Here's how the part is built. I have some questions about the finished solid (model axes, mm). Face numbers are marked on the shaded views. A direction names the side the tool comes from. Round coordinates to 2 decimals unless told otherwise and drop trailing zeros. Order: outer loops, then holes, each group sorted by start corner. A loop starts at its lowest first (then second) coordinate and runs counter-clockwise, first axis right, second up. Notation, with made-up numbers: (23.25, 85) -> (36.25, 85) arc R16 ccw to (36.25, 91) -> close; hole circle Ø3 at (35.5, 74.25). An arc over 180 degrees is marked (long way). One line per item, written item: value.
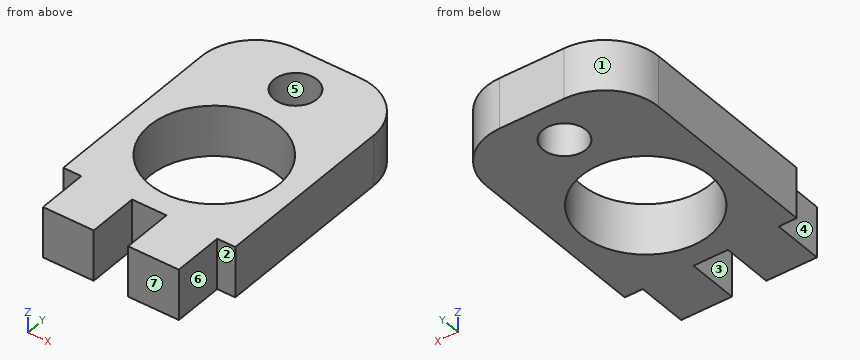
```python
from build123d import *

# Parameters (mm, degrees)
SKETCH1_R           = 3.81
SKETCH1_R_2         = 1.27
BOSS_EXTRUDE1_DEPTH = 2.9972
FILLET1_R           = 3.175


with BuildPart() as part:
    # Sketch1 → Boss-Extrude1 (new body)
    with BuildSketch(Plane.XY):
        Polygon((0, 0), (1.0668, 0), (1.0668, -2.9972), (4.064, -2.9972), (4.064, 0), (6.096, 0), (6.096, -2.9972), (9.0932, -2.9972), (9.0932, 0), (10.16, 0), (10.16, 13.97), (0, 13.97), align=None)
        with Locations(Location((5.08, 5.08, 0), (0, 0, 180))):
            Circle(SKETCH1_R, mode=Mode.SUBTRACT)
        with Locations(Location((5.08, 11.43, 0), (0, 0, 180))):
            Circle(SKETCH1_R_2, mode=Mode.SUBTRACT)
    extrude(amount=BOSS_EXTRUDE1_DEPTH)

    # Fillet1
    fillet1_edges = [part.edges().sort_by_distance(p)[0] for p in [
        (0, 13.97, 1.4986),
        (10.16, 13.97, 1.4986),
    ]]
    fillet(fillet1_edges, radius=FILLET1_R)


solid = part.part
```
Q1. I want a section at C-C on z = 1.75. Write out the boundary of the cut face in (x, y) (3 decimals).
Answers:
outline: (0, 0) -> (1.067, 0) -> (1.067, -2.997) -> (4.064, -2.997) -> (4.064, 0) -> (6.096, 0) -> (6.096, -2.997) -> (9.093, -2.997) -> (9.093, 0) -> (10.16, 0) -> (10.16, 10.795) arc R3.175 ccw to (6.985, 13.97) -> (3.175, 13.97) arc R3.175 ccw to (0, 10.795) -> close; hole circle Ø7.62 at (5.08, 5.08); hole circle Ø2.54 at (5.08, 11.43)
Q2. I want a section at D-D on x = 5. Write out the boundary of the cut face in (y, z).
Answers:
outline: (0, 0) -> (1.27, 0) -> (1.27, 3) -> (0, 3) -> close; (8.89, 0) -> (10.16, 0) -> (10.16, 3) -> (8.89, 3) -> close; (12.7, 0) -> (13.97, 0) -> (13.97, 3) -> (12.7, 3) -> close
Q3. If we mould it in two halves opening along X, with no side actions, what happens to the marked faces 5, 6 and 7? For each: pulls with the +X half, pulls with the -X half, needs draft (parallel to the pull), parting line crosses it, or undercut.
Answers:
face 5: undercut
face 6: pulls with the +X half
face 7: needs draft
Q4. I want a section at A-A on y = -1.5. Write out the boundary of the cut face in (x, z), then the cut area to 3 significant figures.
Answers:
outline: (1.07, 0) -> (4.06, 0) -> (4.06, 3) -> (1.07, 3) -> close; (6.1, 0) -> (9.09, 0) -> (9.09, 3) -> (6.1, 3) -> close
area: 18.0 mm2
Q5. Which directions (+Z, -Z, +X, -X, +Y, -Y) give clear straight access to the entire face, cutting with the end or side of a thin tool? Please do the marked faces 1, 2, 3 and 4.
Answers:
face 1: +Z, -Z, -X, +Y
face 2: +Z, -Z, +X, -Y
face 3: +Z, -Z, -Y
face 4: +Z, -Z, -X, -Y
Q6. I want a section at B-B on x = 7.5. Write out the boundary of the cut face in (y, z).
Answers:
outline: (-3, 0) -> (2.14, 0) -> (2.14, 3) -> (-3, 3) -> close; (8.02, 0) -> (13.93, 0) -> (13.93, 3) -> (8.02, 3) -> close
Q7. For P1, Ø1, axis at x = 5, z = 2, coming from the -Y side; P2, Ø0.9, axis at y = -2, z = 2, coming from the +X side; P3, Ø6, axis at x = 5.08, y = 5.08, coming from the -Z side; P4, Ø0.9, axis at y = -2, z = 1.5, coming from the -X side, each with a flat end and sliding along its axis, tell me the tip position at first contact or that it passes through.
Answers:
P1: y = 0
P2: x = 9.09
P3: through
P4: x = 1.07
Q8. I need wall thicknesses on line 1 along Y through (x, z) = (5.08, 1.1); line 2 along Y through (x, z) = (4, 1.25); line 3 along X through (y, z) = (11.25, 1.6). Which ranges of each line are inside material? Lowest first, please.
Answers:
line 1: 0 to 1.27, 8.89 to 10.16, 12.7 to 13.97
line 2: -3 to 1.43, 8.73 to 10.76, 12.1 to 13.97
line 3: 0.03 to 3.82, 6.34 to 10.13
